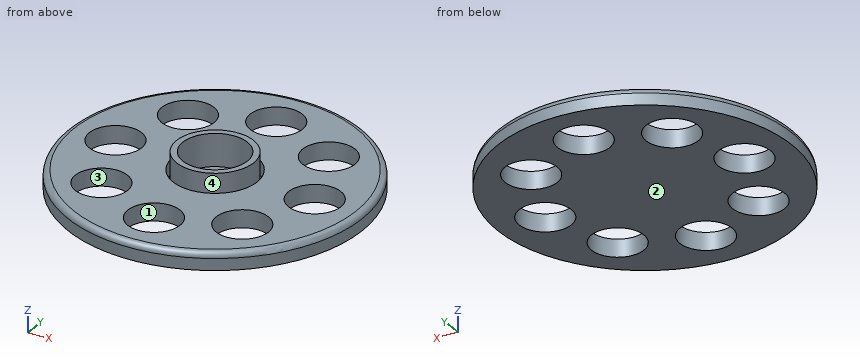
from build123d import *

# Parameters (mm, degrees)
F0_R     = 6.55
F0_R_2   = 5.5
F1_DEPTH = 6
F0_R_3   = 7.15
F2_DEPTH = 0.5
F0_R_4   = 25
F0_R_5   = 4.448453
F3_DEPTH = 3
F4_R     = 1


with BuildPart() as f1:
    # F0 (on Top) → F1 (new body)
    with BuildSketch(Plane.XY):
        Circle(F0_R)
        Circle(F0_R_2, mode=Mode.SUBTRACT)
    extrude(amount=F1_DEPTH)

    # F0 (on Top) → F2 (join)
    with BuildSketch(Plane.XY):
        Circle(F0_R_3)
        Circle(F0_R, mode=Mode.SUBTRACT)
        Circle(F0_R_2)
    extrude(amount=F2_DEPTH)

    # F0 (on Top) → F3 (join)
    with BuildSketch(Plane.XY):
        Circle(F0_R_4)
        with Locations((-12.009858, -12.009858)):
            Circle(F0_R_5, mode=Mode.SUBTRACT)
        with Locations((0, -16.984504)):
            Circle(F0_R_5, mode=Mode.SUBTRACT)
        with Locations((12.009858, -12.009858)):
            Circle(F0_R_5, mode=Mode.SUBTRACT)
        with Locations((-16.984504, 0)):
            Circle(F0_R_5, mode=Mode.SUBTRACT)
        with Locations((-12.009858, 12.009858)):
            Circle(F0_R_5, mode=Mode.SUBTRACT)
        Circle(F0_R_3, mode=Mode.SUBTRACT)
        with Locations((12.009858, 12.009858)):
            Circle(F0_R_5, mode=Mode.SUBTRACT)
        with Locations((16.984504, 0)):
            Circle(F0_R_5, mode=Mode.SUBTRACT)
        with Locations((0, 16.984504)):
            Circle(F0_R_5, mode=Mode.SUBTRACT)
    extrude(amount=F3_DEPTH)

    # F4
    f4_edges = [f1.edges().sort_by_distance(p)[0] for p in [
        (-25, 0, 3),
    ]]
    fillet(f4_edges, radius=F4_R)


solid = f1.part
Build history of the part. All positions in model axes, mm. Face numbers are marked on the shaded views. A direction names the side the tool comes from. Coordinates: 2 decimals unless noted, no trailing zeros. Order: outer loops, then holes, each group sorted by start corner. A loop starts at its lowest first (then second) coordinate and runs counter-clockwise, first axis right, second up. Notation, with made-up numbers: (-36, 49) - (-5, 49) arc R25 cw to (-5, 83) - close; hole circle Ø4 at (56, -31.5). An arc over 180 degrees is marked (long way). Write item = value, one per line. Start each with the question number.
1) Flat gauge pins, fed straight in: pin 1 Ø4.5 at (x, y) = (2.5, 0.5) entering from +Z; pin 2 Ø3 at (x, z) = (-4.5, 2) entering from +Y; pin 3 Ø11.5 at (x, y) = (-16.98, 0) entering from +Z; pin 4 Ø5 at (x, y) = (-13.5, 17) entering from -Z. Where does each tip first touch, or does it go through?
2) 3-axis set-ups, long thin cutter, end or side, ignore diameter. For the marked faces 3 and 4: which of +Z, -Z, +X, -X, +Y, -Y reach the whole face in a straight line?
3) Wall check: line 1 along Y through (x, z) = (0, 1.2); line 2 along X through (y, z) = (1, 2.4); line 3 along X through (y, z) = (-14, 1.85). Give the ranges that are in metal, low to high. Write a range as from..to.
4) Saw through at A-A on x = 0. Write the cut outline in (y, z), then the cut area to 3 significant figures.
5) Two-plate mould, pull along Y, no slides. Class the marked faces 1 and 2: pulls with the +Y half, pulls with the -Y half, needs draft (parallel to the pull), parting line crosses it, or undercut.
6) Saw through at C-C on z = 3.6. Write the cut outline in (x, y), then the cut area to 3 significant figures.
From the geometry:
q1.pin_1 = 0.5
q1.pin_2 = 24.82
q1.pin_3 = 3
q1.pin_4 = 0
q2.face_3 = +Z, -Z
q2.face_4 = +Z
q3.line_1 = -25..-21.43, -12.54..-7.15, -6.55..-5.5, 5.5..6.55, 7.15..12.54, 21.43..25
q3.line_2 = -24.9..-21.32, -12.65..-7.08, -6.47..-5.41, 5.41..6.47, 7.08..12.65, 21.32..24.9
q3.line_3 = -20.71..-15.99, -8.03..-3.3, 3.3..8.03, 15.99..20.71
q4.outline = (-25, 0) - (-21.43, 0) - (-21.43, 3) - (-24, 3) arc R1 ccw to (-25, 2) - close; (-12.54, 0) - (12.54, 0) - (12.54, 3) - (7.15, 3) - (7.15, 0.5) - (6.55, 0.5) - (6.55, 6) - (5.5, 6) - (5.5, 0.5) - (-5.5, 0.5) - (-5.5, 6) - (-6.55, 6) - (-6.55, 0.5) - (-7.15, 0.5) - (-7.15, 3) - (-12.54, 3) - close; (21.43, 0) - (25, 0) - (25, 2) arc R1 ccw to (24, 3) - (21.43, 3) - close
q4.area = 72.0 mm^2
q5.face_1 = undercut
q5.face_2 = needs draft
q6.outline = circle Ø13.1 at (0, 0); hole circle Ø11 at (0, 0)
q6.area = 39.7 mm^2
